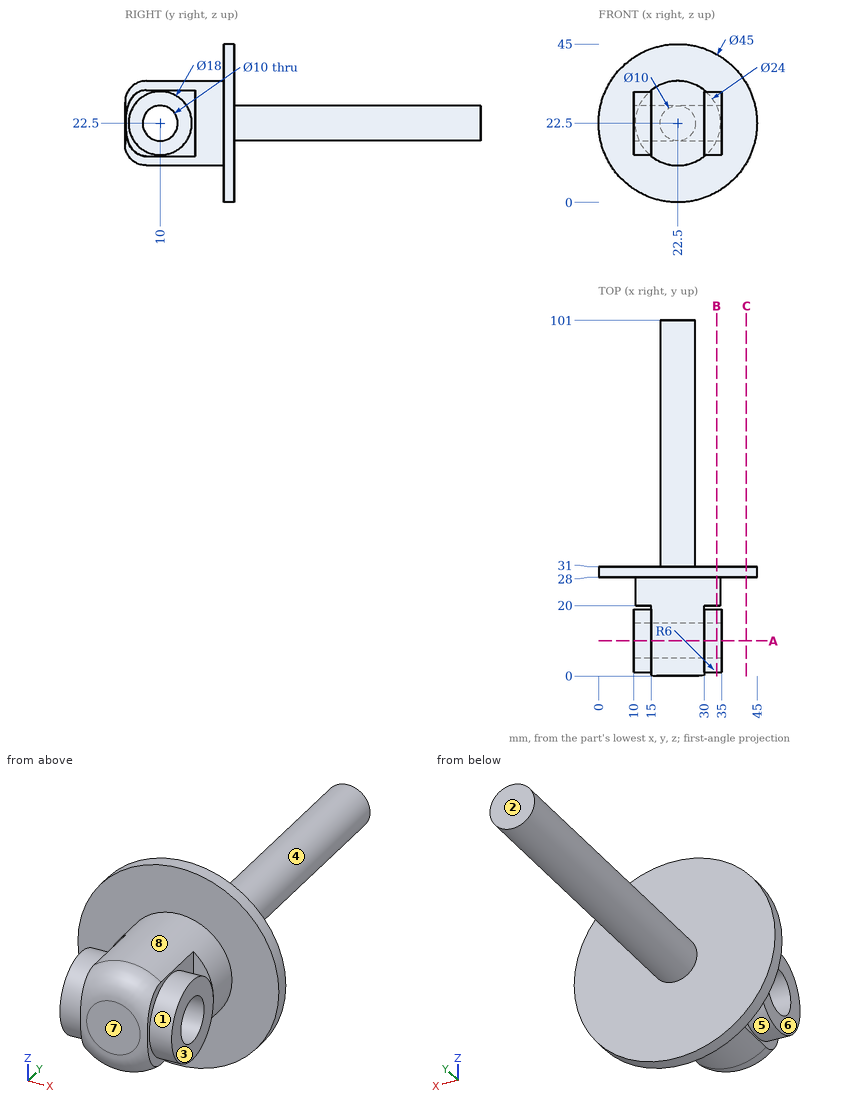
Input: dimensioned drawing with shaded views. Units: mm. Origin: part minimum x, y, z. A direction names the side the tool comes from. Round coordinates to 2 decimals unless told otherwise and drop trailing zeros. Loops run counter-clockwise (first coordinate to the right, second up) from the corner with the lowest first, then second, coordinate; pieces in that order, holes last. Notation, with made-up numbers: (54.25, -23.5) -> (65.25, -23.5) arc R9 ccw to (65.25, -8.5) -> close; hole circle Ø7 at (80, 28). An arc over 180 degrees is marked (long way). Answer as a JSON object with one key per item and string values. Group by question number.
1) Reachability of the marked faces 4, 5, 6, 7 and 8 from +Z, -Z, +X, -X, +Y, -Y: full face, straight path, thin tool, end or side. Return the list, or none.
2) Ray query, L1, parallel to Y at x = 25.5, z = 22.5; L2, parallel to X at y = 16.5, z = 26.5; L3, parallel to Y at x = 18.5, z = 41.5. Return the intervals inside material, ascending.
3) Pin query (flat end, axial travel): pin 1 (10 mm diameter, centred on y = 52.5, z = 16.5, fed in from -X); pin 2 (13.5 mm diameter, centred on x = 31, z = 18, fed in from -Y); pin 3 (1.4 mm diameter, centred on x = 13.5, z = 26, fed in from -Y); pin 4 (8 mm diameter, centred on y = 62, z = 33, fed in from -X). Return the tip coordinate at first contact, or that it passes through.
4) Draft query along Y for the marked faces 1, 2 and 3. Return one class per face: +Y half, -Y half, draft (parallel to the pull), parting line (faces both ways), or undercut.
5) Section query A-A on y = 10. Output: boundary loops of the cut face in (x, z), plus the area to 3 significant figures.
6) Section query B-B on x = 33.5. Output: boundary loops of the cut face in (y, z), plus the area to 3 significant figures.
7) Section query C-C on x = 42. Output: boundary loops of the cut face in (y, z).
Reply:
{
 "1": {"face 4": "+Y", "face 5": "-X", "face 6": "+Z, -Z, -X, -Y", "face 7": "+Z, -Z, +X, -X, -Y", "face 8": "none"},
 "2": {"L1": "y = 0 to 5, 15 to 101", "L2": "x = 10 to 35", "L3": "y = 28 to 31"},
 "3": {"pin 1": "stops at x = 17.6", "pin 2": "stops at y = 0", "pin 3": "stops at y = 1.45", "pin 4": "passes through"},
 "4": {"face 1": "undercut", "face 2": "+Y half", "face 3": "draft"},
 "5": {"outline": "(10, 13.5) -> (15, 13.5) -> (15, 13.13) arc R12 ccw to (30, 13.13) -> (30, 13.5) -> (35, 13.5) -> (35, 17.5) -> (10, 17.5) -> close; (10, 27.5) -> (35, 27.5) -> (35, 31.5) -> (30, 31.5) -> (30, 31.87) arc R12 ccw to (15, 31.87) -> (15, 31.5) -> (10, 31.5) -> close", "area": "265 mm2"},
 "6": {"outline": "circle Ø18 at (10, 22.5); (20, 17.7) -> (28, 17.7) -> (28, 2.87) -> (31, 2.87) -> (31, 42.13) -> (28, 42.13) -> (28, 27.3) -> (20, 27.3) -> close; hole circle Ø10 at (10, 22.5)", "area": "370 mm2"},
 "7": {"outline": "(28, 11.28) -> (31, 11.28) -> (31, 33.72) -> (28, 33.72) -> close"}
}
